Can you work these out from the model? Positions are in its coordinate system, mm. A direction names the side the tool comes from. Coordinates: 2 decimals unless noted, no trailing zeros. Return JSON: item names as keys, results as strings. Group by question number.
1) If I drill on line 1 along Y through (x, z) = (-1.15, 0); line 2 along X through (y, z) = (2.5, 18); line 3 along X through (y, z) = (18, -11.5), over which ranges is the centre line in solid material (lowest first)?
2) For pin 1 Ø2 at (x, z) = (-1.5, -14.5) entering from +Y; pin 2 Ø2 at (x, z) = (-0.5, -0.5) entering from -Y; pin 3 Ø3 at (x, y) = (-2.5, -13.5) entering from -Z, each with a flat end and sliding along its axis, tell me the tip position at first contact or that it passes through.
3) If we mould it in two halves opening along X, with no side actions, what happens to faces 1 (the face through (-4.829, 19.961, -10.382)), 2 (the face through (-1, 17.73, -4.02)), 3 (the face through (0, 14, -11))? For each: pulls with the +X half, pulls with the -X half, needs draft (parallel to the pull), parting line crosses it, or undercut.
4) Which directions (+Z, -Z, +X, -X, +Y, -Y) give clear straight access to the entire face, cutting with the end or side of a thin tool? Please do faces 4 (the face through (-0.51, 16.41, -8.54)), 5 (the face through (-1.507, -12.165, 13.267)), 6 (the face through (-5, 13, -12)).
```python
from build123d import *


with BuildPart() as part:
    # Szkic1 → Obrót1 (revolve)
    with BuildSketch(Plane.XY, mode=Mode.PRIVATE) as obr_t1_sk:
        Polygon((-4.081701013, 20.911565577), (-4.283998784, 20.911565577), (-4.652565061, 22.5), (-5, 22.5), (-5, 17.5), (0, 17.5), (0, 18.5), (-1, 18.5), (-1, 18), (-2, 18), (-2, 22.5), (-2.347434939, 22.5), (-2.899277053, 20.911565577), (-3.101574823, 20.911565577), (-3.415520415, 22.5), (-3.762955354, 22.5), align=None)
    revolve(obr_t1_sk.sketch.rotate(Axis((0, 0, 0), (-1, 0, 0)), 90), axis=Axis((0, 0, 0), (-1, 0, 0)))


solid = part.part
```
Calculated:
{
 "1": {"line 1": "-18 to -17.5, 17.5 to 18", "line 2": "-5 to -2, -1 to 0", "line 3": "-5 to -4.39, -3.99 to -3.19, -2.74 to -2"},
 "2": {"pin 1": "y = 17.9", "pin 2": "y = -18.5", "pin 3": "z = -19.03"},
 "3": {"face 1": "needs draft", "face 2": "undercut", "face 3": "pulls with the +X half"},
 "4": {"face 4": "+X", "face 5": "none", "face 6": "+Z, -Z, -X, +Y, -Y"}
}
